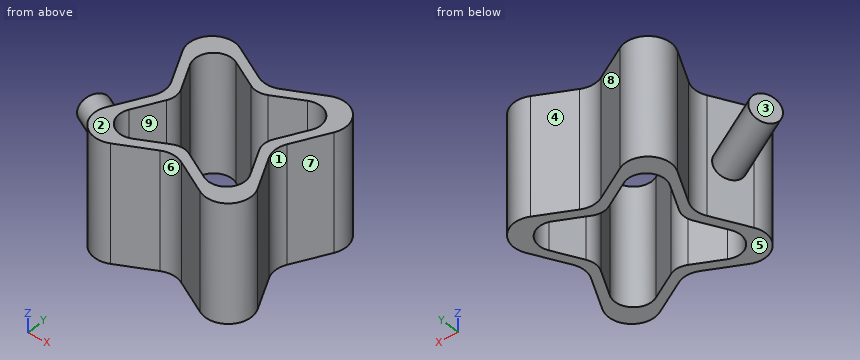
from build123d import *

# Parameters (mm, degrees)
F1_DEPTH = 203.2
F2_R     = 24.4501828069
F3_DEPTH = 127


# Not quite as in the source:
# - ends of sketch curves that miss each other by under 0.0002 mm in the source are joined
# - the program builds the solid bodies; features that only make, move or delete a surface that nothing else refers to are left out


with BuildPart() as f1:
    # F0 (on Top) → F1 (new body)
    with BuildSketch(Plane.XY):
        with BuildLine():
            Line((-18.3351678, 99.7503212), (-76.9148068, 130.3502854))
            ThreePointArc((-76.9148068, 130.3502854), (-123.2518754265, 123.2518754265), (-130.3502933453, 76.9148026497))
            Line((-130.3502933453, 76.9148026497), (-99.7503212, 18.3351678))
            ThreePointArc((-99.7503212, 18.3351678), (-95.25, -1.12567e-05), (-99.7503332097, -18.3351869265))
            Line((-99.7503332097, -18.3351869265), (-130.3502854, -76.9148322))
            ThreePointArc((-130.3502854, -76.9148322), (-123.2518716246, -123.2518792283), (-76.9148130735, -130.3502987903))
            Line((-76.9148130735, -130.3502987903), (-18.3351678, -99.7503466))
            ThreePointArc((-18.3351678, -99.7503466), (1.12567e-05, -95.2500254), (18.3351869265, -99.7503586097))
            Line((18.3351869265, -99.7503586097), (76.9148322, -130.3503108))
            ThreePointArc((76.9148322, -130.3503108), (123.2518754265, -123.2518754265), (130.3503092141, -76.9148330284))
            Line((130.3503092141, -76.9148330284), (99.7503466, -18.3351932))
            ThreePointArc((99.7503466, -18.3351932), (95.25, -1.12567e-05), (99.7503282309, 18.3351773954))
            Line((99.7503282309, 18.3351773954), (130.3503108, 76.9148068))
            ThreePointArc((130.3503108, 76.9148068), (123.2518792283, 123.2518716246), (76.9148226046, 130.3503037691))
            Line((76.9148226046, 130.3503037691), (18.3351932, 99.7503212))
            ThreePointArc((18.3351932, 99.7503212), (1.12567e-05, 95.25), (-18.3351678, 99.7503212))
        make_face()
        with BuildLine():
            ThreePointArc((-104.2802295109, 61.5318322315), (-98.6015083009, 98.6014923815), (-61.5318521865, 104.2802399347))
            Line((-61.5318521865, 104.2802399347), (-14.6681444, 79.8002468))
            ThreePointArc((-14.6681444, 79.8002468), (0, 76.2), (14.6681373897, 79.8002602202))
            Line((14.6681373897, 79.8002602202), (61.5318556, 104.2802334))
            ThreePointArc((61.5318556, 104.2802334), (98.601504143, 98.6014965393), (104.280234956, 61.5318426553))
            Line((104.280234956, 61.5318426553), (79.8002722, 14.6681444))
            ThreePointArc((79.8002722, 14.6681444), (76.2, -1.12567e-05), (79.8002760891, -14.6681677685))
            Line((79.8002760891, -14.6681677685), (104.2802588, -61.5318556))
            ThreePointArc((104.2802588, -61.5318556), (98.6015003412, -98.6015003412), (61.5318626103, -104.2802453798))
            Line((61.5318626103, -104.2802453798), (14.6681444, -79.8002722))
            ThreePointArc((14.6681444, -79.8002722), (0, -76.2000254), (-14.6681373897, -79.8002856202))
            Line((-14.6681373897, -79.8002856202), (-61.5318556, -104.2802588))
            ThreePointArc((-61.5318556, -104.2802588), (-98.6015044991, -98.6014961833), (-104.2802399347, -61.5318521865))
            Line((-104.2802399347, -61.5318521865), (-79.8002468, -14.6681698))
            ThreePointArc((-79.8002468, -14.6681698), (-76.2, -1.12567e-05), (-79.8002602202, 14.6681373897))
            Line((-79.8002602202, 14.6681373897), (-104.2802295109, 61.5318322315))
        make_face(mode=Mode.SUBTRACT)
    extrude(amount=F1_DEPTH)

    # F2 (on face) → F3 (join)
    with BuildSketch(Plane(origin=(-70.8422549592, 37.0055279036, 0), x_dir=(-0.4630021293, -0.8863571674, 0), z_dir=(-0.8863571674, 0.4630021293, 0))):
        with Locations((94.1798388958, 94.7972759604)):
            Circle(F2_R)
    extrude(amount=F3_DEPTH)


solid = f1.part
Geometry check sheet. Reference: the model listing, model coordinates, mm. Face numbers are marked on the shaded views. A direction names the side the tool comes from. Give positions to 0.01 mm unless a question says otherwise; leave off trailing zeros. Order: outer loops, then holes, each group sorted by start corner. A loop starts at its lowest first (then second) coordinate and runs counter-clockwise, first axis right, second up.
1) Draft check along X on the marked faces 1, 2, 3 and 4. Enter one of: released by +X, released by -X, zero draft, split by the parting line, or undercut.
Results are:
face 1: released by +X
face 2: zero draft
face 3: released by -X
face 4: undercut
2) Cross-section at C-C (y = 88). Record the boundary of the cut face in (x, z).
Results are:
outline: (-134.18, 0) - (-105.6, 0) - (-105.6, 203.2) - (-134.18, 203.2) - close; (-30.37, 0) - (30.37, 0) - (30.37, 203.2) - (-30.37, 203.2) - close; (105.6, 0) - (134.18, 0) - (134.18, 203.2) - (105.6, 203.2) - close
3) Gauge pin test, flat ends, axial feed: pin 1 (12 mm diameter, centred on x = -81, y = -1.5, fed in from -Z); pin 2 (1.5 mm diameter, centred on x = 24, z = 171, fed in from -Y); pin 3 (2 mm diameter, centred on y = -32.5, z = 116, fed in from +X); pin 4 (6 mm diameter, centred on x = -87.5, z = 69, fed in from +Y). Record the tip position at first contact, or that the pin passes through.
Results are:
pin 1: stops at z = 0
pin 2: stops at y = -103.1
pin 3: stops at x = 107.67
pin 4: stops at y = 134.56
4) Material ranges on probe 1 along Y at (x, z) = (-79, 43); probe 2 along X at (y, z) = (31.5, 105); probe 3 along Y at (x, z) = (92, 131), recorded low to high.
Results are:
probe 1: y = -131.36 to -107.76, -13.02 to 13.02, 107.76 to 131.36
probe 2: x = -217 to -215.72, -106.63 to -88.59, 88.59 to 106.63
probe 3: y = -134.72 to -103.66, -38.02 to 38.02, 103.66 to 134.72
5) Tool access check on the marked faces 5, 6, 7, 8 and 9. Record the directions out of +Z, -Z, +X, -X, +Y, -Y that give a thin tool (end or side, any length) a straight path to the whole face; none if there is none.
Results are:
face 5: -Z, +X, -X, +Y, -Y
face 6: +Z, -Z, -Y
face 7: +Z, -Z, +X
face 8: +Z, -Z, +Y
face 9: +Z, -Z
6) Cross-section at B-B (x = -37.5). Record the boundary of the cut face in (y, z).
Results are:
outline: (-109.76, 0) - (-91.73, 0) - (-91.73, 203.2) - (-109.76, 203.2) - close; (91.73, 0) - (109.76, 0) - (109.76, 203.2) - (91.73, 203.2) - close
